Input: part model. Units: mm. Frame: model coordinates. A direction names the side the tool comes from. Coordinates: 2 decimals unless noted, no trailing zeros. Order: outer loops, then holes, each group sorted by start corner. A loop starts at its lowest first (then second) coordinate and runs counter-clockwise, first axis right, second up. Notation, with made-up numbers: M 45,45 L 50,45 A16 ccw 50,74 Z; hole C 46,71.5 d8. An arc over 180 degrees is marked long. Answer in a Markdown table with one row per item.
from build123d import *

# Parameters (mm, degrees)
F1_DEPTH = 10
F2_R     = 3
F3_R     = 3
F5_DEPTH = 40
F6_W     = 2
F6_H     = 12
F7_DEPTH = 1
F8_W     = 0.75
F8_H     = 12
F9_DEPTH = 10


with BuildPart() as f1:
    # F0 (on Right) → F1 (new body)
    with BuildSketch(Plane.YZ):
        Polygon((-2.054113, 13.772698), (-8.054113, 13.772698), (-6.429656, 9.711557), (-2.054113, 11.461774), align=None)
        Polygon((3.945887, 13.772698), (-2.054113, 13.772698), (-2.054113, 11.461774), (-2.054113, -1.227302), (3.945887, -16.227302), (3.945887, 12.582935), align=None)
        Polygon((-2.054113, -1.227302), (-2.054113, -16.227302), (3.945887, -16.227302), align=None)
        Polygon((-6.429656, 9.711557), (-8.054113, 13.772698), (-8.054113, -1.227302), (-2.054113, -16.227302), (-2.054113, -1.227302), align=None)
        Polygon((-8.054113, 13.772698), (-14.054113, 13.772698), (-8.054113, -1.227302), align=None)
        Polygon((-8.054113, -1.227302), (-14.054113, 13.772698), (-14.054113, -16.227302), (-8.054113, -16.227302), align=None)
    extrude(amount=F1_DEPTH)

    # F2
    f2_edges = [f1.edges().sort_by_distance(p)[0] for p in [
        (5, -14.054113, 13.772698),
    ]]
    fillet(f2_edges, radius=F2_R)

    # F3
    f3_edges = [f1.edges().sort_by_distance(p)[0] for p in [
        (5, 3.945887, 13.772698),
    ]]
    fillet(f3_edges, radius=F3_R)

    # F4 (on face) → F5 (join)
    with BuildSketch(Plane.XY.offset(13.772698)):
        with BuildLine():
            ThreePointArc((0, -3.804113), (0.53033, -3.584443), (0.75, -3.054113))
            ThreePointArc((0.75, -3.054113), (0.53033, -2.523782), (0, -2.304113))
            Line((0, -2.304113), (0, -3.804113))
        make_face()
        with BuildLine():
            Line((0, -3.804113), (0, -2.304113))
            ThreePointArc((0, -2.304113), (-0.75, -3.054113), (0, -3.804113))
        make_face()
        with BuildLine():
            ThreePointArc((0.75, -7.054113), (0.53033, -6.523782), (0, -6.304113))
            Line((0, -6.304113), (0, -7.804113))
            ThreePointArc((0, -7.804113), (0.53033, -7.584443), (0.75, -7.054113))
        make_face()
        with BuildLine():
            Line((0, -7.804113), (0, -6.304113))
            ThreePointArc((0, -6.304113), (-0.75, -7.054113), (0, -7.804113))
        make_face()
    extrude(amount=F5_DEPTH)

    # F6 (on face) → F7 (join)
    with BuildSketch(Plane.XY.offset(53.772698)):
        with Locations((0, -5.054113)):
            Rectangle(F6_W, F6_H)
    extrude(amount=F7_DEPTH)

    # F8 (on face) → F9 (join)
    with BuildSketch(Plane.XY.offset(54.772698)):
        with Locations((0.625, -5.054113)):
            Rectangle(F8_W, F8_H)
    extrude(amount=F9_DEPTH)


solid = f1.part
1) Reachability of faces 4 (the face through (0.4, -11.054, 58)), 5 (the face through (0, -5, -1)), 6 (the face through (0.4, 0.946, 58)), 7 (the face through (5, -8.054, -9)), 8 (the face through (0.25, -5, 60)) from +Z, -Z, +X, -X, +Y, -Y: full face, straight path, thin tool, end or side. Return the list, or none.
Resolved:
| item | result |
|---|---|
| face 4 | +Z, +X, -X, -Y |
| face 5 | -Z, -X, +Y, -Y |
| face 6 | +Z, +X, -X, +Y |
| face 7 | -Z, +X, -X |
| face 8 | +Z, -X, +Y, -Y |
2) Contact query for flat-ended pins moving along their axis: pin 1 (0.6 mm diameter, centred on x = -0.5, y = -7, fed in from -Z); pin 2 (0.6 mm diameter, centred on x = -0.5, z = 58, fed in from -Y); pin 3 (8 mm diameter, centred on y = -6, z = 60.5, fed in from -X); pin 4 (3 mm diameter, centred on x = 5.5, y = -7.5, fed in from +Z). Output: stop coordinate, or through.
Resolved:
| item | result |
|---|---|
| pin 1 | stops at z = 13.77 |
| pin 2 | passes through |
| pin 3 | stops at x = 0.25 |
| pin 4 | stops at z = 13.77 |
3) Material intervals for probe 1 along Z at (x, y) = (7.25, -1); probe 2 along X at (y, z) = (-6.75, 3.5); probe 3 along X at (y, z) = (-3.5, 56.5), sorted ascending.
Resolved:
| item | result |
|---|---|
| probe 1 | z = -16.23 to 13.77 |
| probe 2 | x = 0 to 10 |
| probe 3 | x = 0.25 to 1 |
4) Cut plane D-D, the plane z = 57. Output: boundary loops of the cut face in (x, y).
Resolved:
| item | result |
|---|---|
| outline | M 0.25,-11.05 L 1,-11.05 L 1,0.95 L 0.25,0.95 Z |
5) Cut plane A-A, the plane x = 7. Output: boundary loops of the cut face in (y, z), and give its area (3 significant figures).
Resolved:
| item | result |
|---|---|
| outline | M -14.05,-16.23 L -8.05,-16.23 L -8.05,-1.23 L -2.05,-16.23 L 3.95,-16.23 L 3.95,10.77 A3 ccw 0.95,13.77 L -11.05,13.77 A3 ccw -14.05,10.77 Z; hole M -6.43,9.71 L -2.05,-1.23 L -2.05,11.46 Z |
| area | 463 mm2 |
6) Cut plane B-B, the plane z = 26. Output: boundary loops of the cut face in (x, y).
Resolved:
| item | result |
|---|---|
| outline | M 0,-6.3 A0.75 ccw long 0.75,-7.05 A0.75 ccw Z; M 0,-2.3 A0.75 ccw long 0.75,-3.05 A0.75 ccw Z |
7) Cut plane C-C, the plane z = -6. Output: boundary loops of the cut face in (x, y), and give its area (3 significant figures).
Resolved:
| item | result |
|---|---|
| outline | M 0,-14.05 L 10,-14.05 L 10,-8.05 L 0,-8.05 Z; M 0,-6.15 L 10,-6.15 L 10,3.95 L 0,3.95 Z |
| area | 161 mm2 |
8) Mould query, pull axis Y, two halves, no side actions, for faces 1 (the face through (5.07, 3.04, 12.92)), 2 (the face through (0, -5, 53.773)), 3 (the face through (1, -5, 59)). Classes: +Y half, -Y half, draft (parallel to the pull), parting line (faces both ways), or undercut.
Resolved:
| item | result |
|---|---|
| face 1 | +Y half |
| face 2 | undercut |
| face 3 | draft |
